For this review, take the finished solid that the model builds, in its own axes (mm). A direction names the side the tool comes from. Give positions to 0.01 mm unless a question says otherwise; leave off trailing zeros. Write each loop counter-clockwise with the first axis right and the second up, starting at its lowest first coordinate (ties: lowest second). Pieces come first, ordered by that corner, then holes.
Q1. We need section C-C (y = 38). Write out the cut boundary in (x, z), then the cut area to 3 significant figures.
Q2. We need section A-A (x = 0). Write out the cut boundary in (y, z).
Q3. Mouldability with a two-part tool opening along X and no side actions: class faces 3 (the flat face through (10, 61.9, 10)), 4 (the flat face through (0, 4, 22.405)), 5 (the cylindrical face through (-0.867, 77.274, 3.905)), 6 (the cylindrical face through (8.79, 64.18, 8.89)) as released by +X, released by -X, zero draft, split by the parting line, or undercut.
Q4. Insertion check: P1, Ø0.9, axis at x = 9.5, z = -10, coming from the +Y side; P2, Ø3.5, axis at x = -10, z = 9, coming from the +Y side; P3, Ø5, axis at y = 48, z = -7.5, coming from the +X side. Each pin has a flat end and moves straight along its axis. Give the tip position at first contact, or say it passes through.
Q5. We need section B-B (z = 0). Write out the cut boundary in (x, y), then the cut area to 3 significant figures.
Q6. We need section D-D (x = -14). Write out the cut boundary in (y, z), then the cut area to 3 significant figures.
Q7. For line 1 (X direction, y = 66, z = 10.5); line 2 (Z direction, x = 0.5, y = 24); line 3 (Y direction, x = 12, z = 13.5), list the stretches that pass through material, from the lowest coordinate up.
Q8. Machinability: for faces 1 (the cylindrical face through (8.4, 64.18, -9.97)), 2 (the flat face through (0, 86.4, 0)), which of the approach directions +Z, -Z, +X, -X, +Y, -Y give a long, thin tool a straight path to every point of the face, cutting with its end or side? Answer none if there is none.
```python
from build123d import *

# Parameters (mm, degrees)
SKETCH1_R           = 18.01
SKETCH1_R_2         = 11
SKETCH1_R_3         = 1.5
SKETCH1_R_4         = 4
BOSS_EXTRUDE1_DEPTH = 44.6
BOSS_EXTRUDE2_START = 44.6
SKETCH1_3_R         = 18.01
SKETCH1_3_R_2       = 11
SKETCH1_3_R_3       = 1.5
SKETCH1_3_R_4       = 4
BOSS_EXTRUDE2_DEPTH = 21.8
BOSS_EXTRUDE3_START = 66.4
SKETCH1_4_R         = 11
SKETCH1_4_R_2       = 4
BOSS_EXTRUDE3_DEPTH = 2
CUT_EXTRUDE1_START  = 66.4
SKETCH1_5_R         = 1.5
CUT_EXTRUDE1_DEPTH  = 4.5
BOSS_EXTRUDE4_START = 66.4
SKETCH1_6_R         = 4
BOSS_EXTRUDE4_DEPTH = 20
SKETCH1_7_W         = 12.459329624
SKETCH1_7_H         = 1.245276847
BOSS_EXTRUDE5_DEPTH = 9


with BuildPart() as part:
    # Sketch1 → Boss-Extrude1 (new body)
    with BuildSketch(Plane(origin=(0, 0, 0), x_dir=(1, 0, 0), z_dir=(0, 1, 0))):
        Polygon((-17.084609899, 21.16), (-21.16, 16.798777214), (-21.16, -17.201222786), (-16.923568895, -21.16), (-6.229664812, -21.16), (6.229664812, -21.16), (17.310192914, -21.16), (21.16, -17.040181782), (21.16, 17.193580027), (16.915390101, 21.16), align=None)
        Circle(SKETCH1_R, mode=Mode.SUBTRACT)
        Circle(SKETCH1_R)
        Circle(SKETCH1_R_2, mode=Mode.SUBTRACT)
        with Locations((-9.899494937, 9.899494937)):
            Circle(SKETCH1_R_3, mode=Mode.SUBTRACT)
        with Locations((-9.899494937, -9.899494937)):
            Circle(SKETCH1_R_3, mode=Mode.SUBTRACT)
        with Locations((9.899494937, -9.899494937)):
            Circle(SKETCH1_R_3, mode=Mode.SUBTRACT)
        with Locations((9.899494937, 9.899494937)):
            Circle(SKETCH1_R_3, mode=Mode.SUBTRACT)
        Circle(SKETCH1_R_2)
        Circle(SKETCH1_R_4, mode=Mode.SUBTRACT)
        with Locations((9.899494937, 9.899494937)):
            Circle(SKETCH1_R_3)
        with Locations((9.899494937, -9.899494937)):
            Circle(SKETCH1_R_3)
        with Locations((-9.899494937, -9.899494937)):
            Circle(SKETCH1_R_3)
        with Locations((-9.899494937, 9.899494937)):
            Circle(SKETCH1_R_3)
        Circle(SKETCH1_R_4)
    extrude(amount=BOSS_EXTRUDE1_DEPTH)

    # Sketch1<3> → Boss-Extrude2 (add)
    with BuildSketch(Plane(origin=(0, 0, 0), x_dir=(1, 0, 0), z_dir=(0, 1, 0)).offset(BOSS_EXTRUDE2_START)):
        Circle(SKETCH1_3_R)
        Circle(SKETCH1_3_R_2, mode=Mode.SUBTRACT)
        with Locations((-9.899494937, 9.899494937)):
            Circle(SKETCH1_3_R_3, mode=Mode.SUBTRACT)
        with Locations((-9.899494937, -9.899494937)):
            Circle(SKETCH1_3_R_3, mode=Mode.SUBTRACT)
        with Locations((9.899494937, -9.899494937)):
            Circle(SKETCH1_3_R_3, mode=Mode.SUBTRACT)
        with Locations((9.899494937, 9.899494937)):
            Circle(SKETCH1_3_R_3, mode=Mode.SUBTRACT)
        Circle(SKETCH1_3_R_2)
        Circle(SKETCH1_3_R_4, mode=Mode.SUBTRACT)
        with Locations((-9.899494937, -9.899494937)):
            Circle(SKETCH1_3_R_3)
        with Locations((9.899494937, -9.899494937)):
            Circle(SKETCH1_3_R_3)
        with Locations((9.899494937, 9.899494937)):
            Circle(SKETCH1_3_R_3)
        with Locations((-9.899494937, 9.899494937)):
            Circle(SKETCH1_3_R_3)
        Circle(SKETCH1_3_R_4)
    extrude(amount=BOSS_EXTRUDE2_DEPTH)

    # Sketch1<4> → Boss-Extrude3 (add)
    with BuildSketch(Plane(origin=(0, 0, 0), x_dir=(1, 0, 0), z_dir=(0, 1, 0)).offset(BOSS_EXTRUDE3_START)):
        Circle(SKETCH1_4_R)
        Circle(SKETCH1_4_R_2, mode=Mode.SUBTRACT)
        Circle(SKETCH1_4_R_2)
    extrude(amount=BOSS_EXTRUDE3_DEPTH)

    # Sketch1<5> → Cut-Extrude1 (cut)
    with BuildSketch(Plane(origin=(0, 0, 0), x_dir=(1, 0, 0), z_dir=(0, 1, 0)).offset(CUT_EXTRUDE1_START)):
        with Locations((9.899494937, -9.899494937)):
            Circle(SKETCH1_5_R)
        with Locations((9.899494937, 9.899494937)):
            Circle(SKETCH1_5_R)
        with Locations((-9.899494937, 9.899494937)):
            Circle(SKETCH1_5_R)
        with Locations((-9.899494937, -9.899494937)):
            Circle(SKETCH1_5_R)
    extrude(amount=-CUT_EXTRUDE1_DEPTH, mode=Mode.SUBTRACT)

    # Sketch1<6> → Boss-Extrude4 (add)
    with BuildSketch(Plane(origin=(0, 0, 0), x_dir=(1, 0, 0), z_dir=(0, 1, 0)).offset(BOSS_EXTRUDE4_START)):
        Circle(SKETCH1_6_R)
    extrude(amount=BOSS_EXTRUDE4_DEPTH)

    # Sketch1<7> → Boss-Extrude5 (add)
    with BuildSketch(Plane(origin=(0, 0, 0), x_dir=(1, 0, 0), z_dir=(0, 1, 0))):
        with Locations((0, -21.782638423)):
            Rectangle(SKETCH1_7_W, SKETCH1_7_H)
    extrude(amount=BOSS_EXTRUDE5_DEPTH)


solid = part.part
```
Computed:
1. outline: (-21.16, -16.8) - (-17.08, -21.16) - (16.92, -21.16) - (21.16, -17.19) - (21.16, 17.04) - (17.31, 21.16) - (-16.92, 21.16) - (-21.16, 17.2) - close
1. area: 1,760 mm2
2. outline: (0, -21.16) - (44.6, -21.16) - (44.6, -18.01) - (66.4, -18.01) - (66.4, -11) - (68.4, -11) - (68.4, -4) - (86.4, -4) - (86.4, 4) - (68.4, 4) - (68.4, 11) - (66.4, 11) - (66.4, 18.01) - (44.6, 18.01) - (44.6, 21.16) - (9, 21.16) - (9, 22.41) - (0, 22.41) - close
3. face 3: undercut
3. face 4: zero draft
3. face 5: split by the parting line
3. face 6: undercut
4. P1: stops at y = 61.9
4. P2: stops at y = 66.4
4. P3: stops at x = 17.3
5. outline: (-21.16, 0) - (21.16, 0) - (21.16, 44.6) - (18.01, 44.6) - (18.01, 66.4) - (11, 66.4) - (11, 68.4) - (4, 68.4) - (4, 86.4) - (-4, 86.4) - (-4, 68.4) - (-11, 68.4) - (-11, 66.4) - (-18.01, 66.4) - (-18.01, 44.6) - (-21.16, 44.6) - close
5. area: 2,860 mm2
6. outline: (0, -21.16) - (44.6, -21.16) - (44.6, -11.33) - (66.4, -11.33) - (66.4, 11.33) - (44.6, 11.33) - (44.6, 21.16) - (0, 21.16) - close
6. area: 2,380 mm2
7. line 1: x = -14.63 to -11.27, -8.52 to 8.52, 11.27 to 14.63
7. line 2: z = -21.16 to 21.16
7. line 3: y = 0 to 44.6
8. face 1: +Y
8. face 2: +Z, -Z, +X, -X, +Y
